Geometry: final body of the model. Coordinates: model frame, mm. A direction names the side the tool comes from. Give positions to 0.01 mm unless a question says otherwise; leave off trailing zeros. Order: outer loops, then holes, each group sorted by start corner. A loop starts at its lowest first (then second) coordinate and runs counter-clockwise, first axis right, second up. Notation, with made-up numbers: (63.25, 45.5) -> (72.25, 45.5) arc R24 ccw to (72.25, 62.5) -> close; hole circle Ø10 at (89, 47). An arc over 180 degrees is marked (long way). One line per question, with ' | ' between items. Start each with the question number.
(1) Section B-B (x = 5). Return loops of the section in (y, z).
(2) Section A-A (y = -2). Return loops of the section in (x, z) (3 decimals).
(3) Section D-D (y = 6.75). Return loops of the section in (x, z), then the cut area to 3 significant figures.
(4) First-contact query: pin 1 Ø1.3 at (y, z) = (-1, 0.5) entering from -X (3 decimals); pin 2 Ø1.3 at (y, z) = (-1, 0.5) entering from +X (3 decimals); pin 3 Ø0.6 at (x, y) = (5.5, -0.5) entering from -Z. Flat tips, straight axial feed; report the tip coordinate or a pass-through.
(5) Ray query, L1, parallel to Z at x = 5.75, y = -1; L2, parallel to Z at x = 4.5, y = 6.5; L3, parallel to Y at x = 4.5, z = 1.75. Return the intervals inside material, ascending.
(6) Set-up query: faces 1 (the face through (3, 3, 2.3)), 2 (the face through (3.3, 6.5, 0.52)), 3 (the face through (3.24, 0.07, 0.49)). Return all of +Z, -Z, +X, -X, +Y, -Y with unobstructed straight access to the full face (end or side cutting, diameter ignored); none if empty.
(7) Section C-C (x = 3.5). Return loops of the section in (y, z).
```python
from build123d import *

# Parameters (mm, degrees)
SKETCH1_W           = 6.58
SKETCH1_H           = 6.1
BOSS_EXTRUDE1_DEPTH = 2.3
DRAFT1_ANGLE        = -8
CHAMFER1_SIZE       = 1
CHAMFER1_SIZE2      = 0.140540835
BOSS_EXTRUDE2_DEPTH = 0.52
EXTRUDE_THIN1_DEPTH = 0.38
SKETCH4_W           = 0.17
SKETCH4_H           = 0.83
EXTRUDE_THIN2_DEPTH = 0.38


with BuildPart() as part:
    # Sketch1 → Boss-Extrude1 (new body)
    with BuildSketch(Plane.XY):
        with Locations((3.29, 3.05)):
            Rectangle(SKETCH1_W, SKETCH1_H)
    extrude(amount=BOSS_EXTRUDE1_DEPTH)

    # Draft1
    draft1_faces = [part.faces().sort_by_distance(p)[0] for p in [
        (3.29, 6.1, 1.15),
    ]]
    draft(draft1_faces, Plane(origin=(0, 0, 0), x_dir=(-1, 0, 0), z_dir=(0, 0, -1)), DRAFT1_ANGLE)

    # Chamfer1
    chamfer1_edges = [part.edges().sort_by_distance(p)[0] for p in [
        (3.29, 0, 0),
        (3.29, 0, 2.3),
    ]]
    chamfer1_side = [part.faces().sort_by_distance(p)[0] for p in [
        (3.29, 0, 1.15),
    ]]
    chamfer(chamfer1_edges, length=CHAMFER1_SIZE, length2=CHAMFER1_SIZE2, reference=chamfer1_side[0])

    # Sketch2 → Boss-Extrude2 (add)
    with BuildSketch(Plane.XY):
        Polygon((0.61, 5.77675608), (5.97, 5.77675608), (5.97, 6.1), (5.97, 7.3), (5.29, 7.3), (5.29, 6.9), (1.29, 6.9), (1.29, 7.3), (0.61, 7.3), (0.61, 6.1), align=None)
    extrude(amount=BOSS_EXTRUDE2_DEPTH)

    # Sketch3 → Extrude-Thin1 (add, symmetric)
    with BuildSketch(Plane(origin=(5.575, 0, 0), x_dir=(0, 0, -1), z_dir=(1, 0, 0))):
        with BuildLine():
            Line((-1, 0), (-1, -1.21))
            ThreePointArc((-1, -1.21), (-0.912132034, -1.422132034), (-0.7, -1.51))
            Line((-0.7, -1.51), (-0.3, -1.51))
            ThreePointArc((-0.3, -1.51), (-0.087867966, -1.597867966), (0, -1.81))
            Line((0, -1.81), (0, -2.61))
            Line((0, -2.61), (-0.17, -2.61))
            Line((-0.17, -2.61), (-0.17, -1.81))
            ThreePointArc((-0.17, -1.81), (-0.208076118, -1.718076118), (-0.3, -1.68))
            Line((-0.3, -1.68), (-0.7, -1.68))
            ThreePointArc((-0.7, -1.68), (-1.032340187, -1.542340187), (-1.17, -1.21))
            Line((-1.17, -1.21), (-1.17, 0))
            Line((-1.17, 0), (-1, 0))
        make_face()
    extrude_thin1 = extrude(amount=EXTRUDE_THIN1_DEPTH, both=True)

    # Mirror1: Extrude-Thin1 across plane
    add(extrude_thin1.mirror(Plane(origin=(3.29, 0, 0), x_dir=(0, 0, 1), z_dir=(1, 0, 0))))

    # Sketch4 → Extrude-Thin2 (add, symmetric)
    with BuildSketch(Plane(origin=(3.29, 0, 0), x_dir=(0, 0, -1), z_dir=(1, 0, 0))):
        with Locations((-1.085, -0.415)):
            Rectangle(SKETCH4_W, SKETCH4_H)
    extrude(amount=EXTRUDE_THIN2_DEPTH, both=True)


solid = part.part
```
Response:
1) outline: (0, 1) -> (0.14, 0) -> (6.9, 0) -> (6.9, 0.52) -> (6.03, 0.52) -> (5.78, 2.3) -> (0.14, 2.3) -> (0, 1.3) -> close
2) outline: (0.625, 0) -> (1.385, 0) -> (1.385, 0.17) -> (0.625, 0.17) -> close; (5.195, 0) -> (5.955, 0) -> (5.955, 0.17) -> (5.195, 0.17) -> close
3) outline: (0.61, 0) -> (5.97, 0) -> (5.97, 0.52) -> (0.61, 0.52) -> close | area: 2.79 mm^2
4) pin 1: stops at x = 0.625 | pin 2: stops at x = 5.955 | pin 3: stops at z = 1
5) L1: z = 1 to 1.17 | L2: z = 0 to 0.52 | L3: y = 0.06 to 5.85
6) face 1: +Z, +X, -X, +Y, -Y | face 2: +Z, +X, -X, +Y | face 3: -Z, +X, -X
7) outline: (-0.83, 1) -> (0, 1) -> (0.14, 0) -> (6.9, 0) -> (6.9, 0.52) -> (6.03, 0.52) -> (5.78, 2.3) -> (0.14, 2.3) -> (0, 1.3) -> (0, 1.17) -> (-0.83, 1.17) -> close
